from build123d import *

# Parameters (mm, degrees)
BOX005014_W     = 3
BOX005014_H     = 12
BOX005014_DEPTH = 2
BOX005012_W     = 3
BOX005012_H     = 2.7
BOX005012_DEPTH = 2.7
BOX005011_W     = 3
BOX005011_H     = 2.7
BOX005011_DEPTH = 2.7
BOX005009_W     = 35
BOX005009_H     = 16
BOX005009_DEPTH = 18.5


with BuildPart() as krychle013:
    # Box005014 → Box005014 (new body)
    with BuildSketch(Plane(origin=(20, 77, -26), x_dir=(1, 0, 0), z_dir=(0, 0, 1))):
        with Locations((1.5, 6)):
            Rectangle(BOX005014_W, BOX005014_H)
    extrude(amount=BOX005014_DEPTH)


with BuildPart() as krychle011:
    # Box005012 → Box005012 (new body)
    with BuildSketch(Plane(origin=(-5, 88.4, -45.8), x_dir=(1, 0, 0), z_dir=(0, 0, 1))):
        with Locations((1.5, 1.35)):
            Rectangle(BOX005012_W, BOX005012_H)
    extrude(amount=BOX005012_DEPTH)


with BuildPart() as krychle010:
    # Box005011 → Box005011 (new body)
    with BuildSketch(Plane(origin=(-5, 75, -45.8), x_dir=(1, 0, 0), z_dir=(0, 0, 1))):
        with Locations((1.5, 1.35)):
            Rectangle(BOX005011_W, BOX005011_H)
    extrude(amount=BOX005011_DEPTH)


with BuildPart() as obj1:
    # Box005009 → Box005009 (new body)
    with BuildSketch(Plane(origin=(-5, 75, -44), x_dir=(1, 0, 0), z_dir=(0, 0, 1))):
        with Locations((17.5, 8)):
            Rectangle(BOX005009_W, BOX005009_H)
    extrude(amount=BOX005009_DEPTH)

    # Cut: cut Krychle010
    add(krychle010.part, mode=Mode.SUBTRACT)

    # Cut001: cut Krychle011
    add(krychle011.part, mode=Mode.SUBTRACT)

    # Cut002: cut Krychle013
    add(krychle013.part, mode=Mode.SUBTRACT)


solid = obj1.part
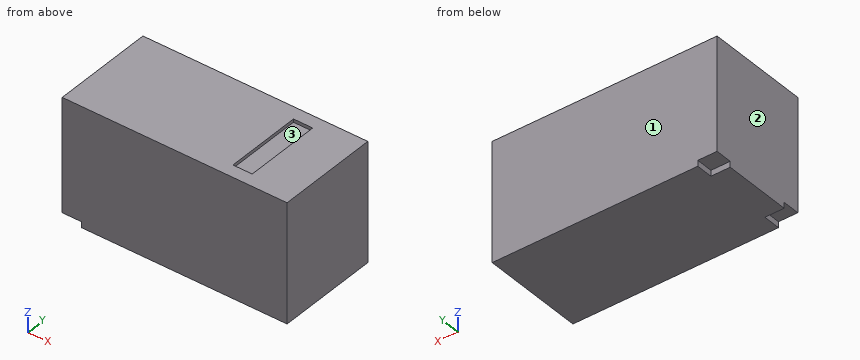
Can you work these out from the model? Positions are in its coordinate system, mm. Face numbers are marked on the shaded views. Coordinates: 2 decimals unless noted, no trailing zeros. Write each loop counter-clockwise with the first axis right and the second up, starting at its lowest first coordinate (ties: lowest second). Pieces come first, ordered by that corner, then holes. Notation, with made-up numbers: (-24, 83) - (4, 83) arc R13 cw to (4, 96) - close; hole circle Ø4 at (71, 81.25). An arc over 180 degrees is marked (long way). Return JSON: item names as keys, results as strings. Group by question number.
Item 1: If we section it at A-A (x = 21): Write out the boundary of the cut face in (y, z).
Item 2: I'm going to push flat-ended pins straight in: pin 1 Ø0.5 at (x, z) = (-3, -43.5) entering from +Y; pin 2 Ø1.5 at (x, y) = (21.5, 84.5) entering from +Z; pin 3 Ø0.5 at (y, z) = (76, -43.5) entering from -X. Where does each tip first touch, or does it pass through?
Item 3: We'd pull the mould along X, two halves only. Please class the marked faces 1, 2 and 3: pulls with the +X half, pulls with the -X half, needs draft (parallel to the pull), parting line crosses it, or undercut.
Return value:
{
 "1": {"outline": "(75, -44) - (91, -44) - (91, -25.5) - (89, -25.5) - (89, -26) - (77, -26) - (77, -25.5) - (75, -25.5) - close"},
 "2": {"pin 1": "stops at y = 88.4", "pin 2": "stops at z = -26", "pin 3": "stops at x = -2"},
 "3": {"face 1": "needs draft", "face 2": "pulls with the -X half", "face 3": "undercut"}
}
